Could you check a few things on this model? Use its own coordinates, in mm. Round coordinates to 2 decimals unless told otherwise and drop trailing zeros. Loops run counter-clockwise (first coordinate to the right, second up) from the corner with the lowest first, then second, coordinate; pieces in that order, holes last. Notation, with made-up numbers: M -10,44.25 L 30,44.25 A33 cw 30,79.25 Z; hole C 55,-12 d11. An arc over 180 degrees is marked long. Return JSON: item names as keys, results as strings. Group by question number.
Autodesk Inventor part; units mm, degrees
ref_plane "YZ Plane" through (0, 0, 0) normal (1, 0, 0) x (0, 1, 0)
ref_plane "XZ Plane" through (0, 0, 0) normal (0, 1, 0) x (-1, 0, 0)
ref_plane "XY Plane" through (0, 0, 0) normal (0, 0, 1) x (1, 0, 0)
sketch "Sketch1" plane through (0, 0, 0) normal (0, 0, 1) x (1, 0, 0)
  line L0 (-15, 7) -> (15, 7)
  line L1 (15, 7) -> (15, -7)
  line L2 (15, -7) -> (-15, -7)
  line L3 (-15, -7) -> (-15, 7)
  line L4 (-15, 7) -> (-23, 7)
  line L5 (-23, 7) -> (-23, -7)
  line L6 (-23, -7) -> (-15, -7)
  line L7 (-15, -7) -> (-15, 7)
  line L8 (15, 7) -> (23, 7)
  line L9 (23, 7) -> (23, -7)
  line L10 (23, -7) -> (15, -7)
  line L11 (15, -7) -> (15, 7)
  line L12 (-23, 0) -> (23, 0) construction
  circle A0 centre (-19, 0) radius 2.25
  circle A1 centre (19, 0) radius 2.25
  line L13 (0, 7) -> (0, -7) construction
  line L14 (-8.5, 7) -> (8.5, 7)
  line L15 (8.5, 7) -> (8.5, 1)
  line L16 (8.5, 1) -> (-8.5, 1)
  line L17 (-8.5, 1) -> (-8.5, 7)
  point P0 (0, 0)
  point P1 (0, 0)
  point P2 (0, 7)
  point P3 (0, 0)
  dimension "d0" = 14
  dimension "d1" = 30
  dimension "d2" = 4.5
  dimension "d3" = 4.5
  dimension "d4" = 4
  dimension "d5" = 4
  dimension "d6" = 4
  dimension "d7" = 4
  dimension "d10" = 17
  dimension "d11" = 6
extrude "Extrusion1" add sketch "Sketch1" along normal blind 1.5 contours L0 L17 L16 L15 L1 L2 L3 | L3 L6 L5 L4 | L1 L8 L9 L10
properties part number "MotorBar"
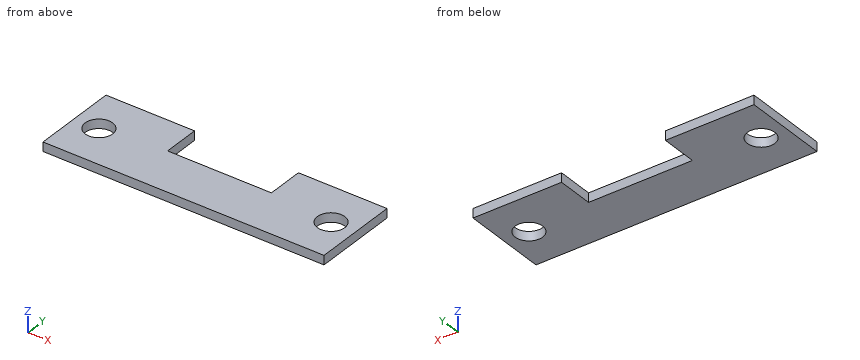
1. If we section it at B-B, the plane x = 19: Please give me the cut outline in (y, z).
2. I need wall thicknesses on probe 1 along Y at (x, z) = (-19, 0.8); probe 2 along X at (y, z) = (0.5, 0.2); probe 3 along X at (y, z) = (2.75, 0.7). Which ranges of each line are inside material? Lowest first, please.
3. If we section it at A-A, the plane y = 0: Please give me the cut outline in (x, z), then the cut area to 3 significant figures.
4. If we section it at D-D, the plane x = -18.5: Please give me the cut outline in (y, z), then the cut area to 3 significant figures.
5. If we section it at C-C, the plane z = 0.9: Please give me the cut outline in (x, y).
6. I'm going to push a flat-ended pin straight in: pin 1 Ø7 at (x, y) = (-19, 0) entering from -Z. Where does the tip first touch, or does it pass through?
Geometry results:
{
 "1": {"outline": "M -7,0 L -2.25,0 L -2.25,1.5 L -7,1.5 Z; M 2.25,0 L 7,0 L 7,1.5 L 2.25,1.5 Z"},
 "2": {"probe 1": "-7 to -2.25, 2.25 to 7", "probe 2": "-23 to -21.19, -16.81 to 16.81, 21.19 to 23", "probe 3": "-23 to -8.5, 8.5 to 23"},
 "3": {"outline": "M -23,0 L -21.25,0 L -21.25,1.5 L -23,1.5 Z; M -16.75,0 L 16.75,0 L 16.75,1.5 L -16.75,1.5 Z; M 21.25,0 L 23,0 L 23,1.5 L 21.25,1.5 Z", "area": "55.5 mm^2"},
 "4": {"outline": "M -7,0 L -2.19,0 L -2.19,1.5 L -7,1.5 Z; M 2.19,0 L 7,0 L 7,1.5 L 2.19,1.5 Z", "area": "14.4 mm^2"},
 "5": {"outline": "M -23,-7 L 23,-7 L 23,7 L 8.5,7 L 8.5,1 L -8.5,1 L -8.5,7 L -23,7 Z; hole C -19,0 d4.5; hole C 19,0 d4.5"},
 "6": {"pin 1": "z = 0"}
}
